Part print with two shaded views. Sizes in mm from the minimum x, y, z corner. Give positions to 0.01 mm unless a question says otherwise; leave off trailing zeros. Loops run counter-clockwise (first coordinate to the right, second up) from the corner with the lowest first, then second, coordinate; pieces in that order, holes last. Notation, with made-up numbers: (62.25, -11) -> (69.25, -11) arc R25 ccw to (69.25, 22) -> close; hole circle Ø8 at (-6.5, 54.25). An arc over 180 degrees is marked (long way). One line per question, with ' | ' between items.
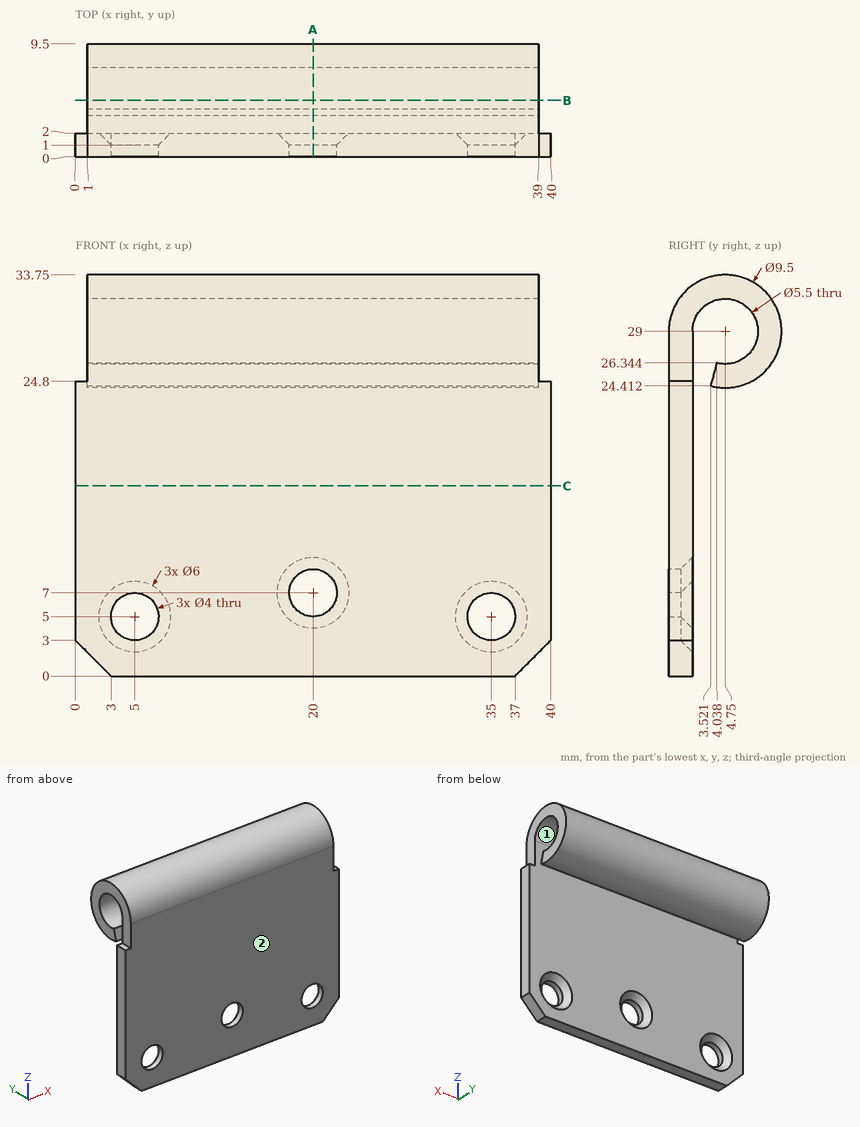
1) Drill centre lines: line 1 (Z direction, x = 29.5, y = 4.75); line 2 (Y direction, x = 2, z = 17.5); line 3 (Y direction, x = 24.5, z = 27) (1 decimal). Where is each one in solid material? Low to high.
Found:
line 1: 24.25 to 26.25, 31.75 to 33.75 | line 2: 0 to 2 | line 3: 0 to 2, 6.6 to 9.1
2) Saw through at A-A (x = 20). Give the cut face in (y, z).
Found:
outline: (0, 0) -> (2, 0) -> (2, 4) -> (1, 5) -> (0, 5) -> close; (0, 9) -> (1, 9) -> (2, 10) -> (2, 29) arc R2.75 cw (long way) to (4.04, 26.34) -> (3.52, 24.41) arc R4.75 ccw (long way) to (0, 29) -> close
3) Saw through at C-C (z = 16). Give the cut face in (x, y).
Found:
outline: (0, 0) -> (40, 0) -> (40, 2) -> (0, 2) -> close
4) Pin check, flat tips, straight feed: P1, Ø6.5, axis at x = 35, z = 5, coming from the +Y side; P2, Ø0.5, axis at x = 39.5, y = 1, coming from the +Z side. Stop position of each tip, or through.
Found:
P1: y = 2 | P2: z = 24.8
5) Pull direction Y, two halves, no side cores. Call the marked faces 1 and 2: pulls with the +Y half, pulls with the -Y half, needs draft (parallel to the pull), parting line crosses it, or undercut.
Found:
face 1: undercut | face 2: pulls with the -Y half
6) Saw through at B-B (y = 4.75). Give the cut face in (x, z), and give its area (3 significant figures).
Found:
outline: (1, 24.25) -> (39, 24.25) -> (39, 26.25) -> (1, 26.25) -> close; (1, 31.75) -> (39, 31.75) -> (39, 33.75) -> (1, 33.75) -> close | area: 152 mm2
